Could you check a few things on this model? Use its own coordinates, in mm. Face numbers are marked on the shaded views. A direction names the side the tool comes from. Give positions to 0.01 mm unless a question says otherwise; leave off trailing zeros. Loops run counter-clockwise (first coordinate to the right, second up) from the corner with the lowest first, then second, coordinate; pieces in that order, holes last. Notation, with made-up numbers: (31, 28) -> (37, 28) arc R23 cw to (37, 62) -> close; hole circle Ø11 at (-7, 80.25). An arc over 180 degrees is marked (long way). Write each question's results on one line, items separated by ' | '. Start each with the question number.
Q1. If we section it at D-D, the plane x = 54.5: List the corners of the cut face in (y, z) for me, plus the area to 3 significant figures.
Q2. If we section it at A-A, the plane x = 0: List the corners of the cut face in (y, z) for me, plus the area to 3 significant figures.
Q3. If we section it at C-C, the plane y = 12: List the corners of the cut face in (x, z) for me.
Q4. If we section it at B-B, the plane z = -33: List the corners of the cut face in (x, y) for me.
Q5. Which directions (+Z, -Z, +X, -X, +Y, -Y) give clear straight access to the entire face, cutting with the end or side of a thin tool? Please do the marked faces 4, 5, 6 and 7.
Q6. Will these pins go through, and if not, where does the flat tip stop? P1, Ø11, axis at x = 1, z = 3, coming from the -Y side; P2, Ø1, axis at y = 19.5, z = -10.5, coming from the -X side; P3, Ø12, axis at y = 20.5, z = -5, coming from the +X side; P4, Ø4, axis at x = 1.5, z = -1.5, coming from the +Y side.
Q7. If I drill on line 1 along X through (y, z) = (41, 0); line 2 along Z through (x, y) = (55, 40.5); line 3 along Z through (x, y) = (57, 75), over which ranges is the centre line in solid material (lowest first)?
Q8. We'd pull the mould along Z, two halves only. Please class the marked faces 1, 2 and 3: released by +Z, released by -Z, zero draft, split by the parting line, or undercut.
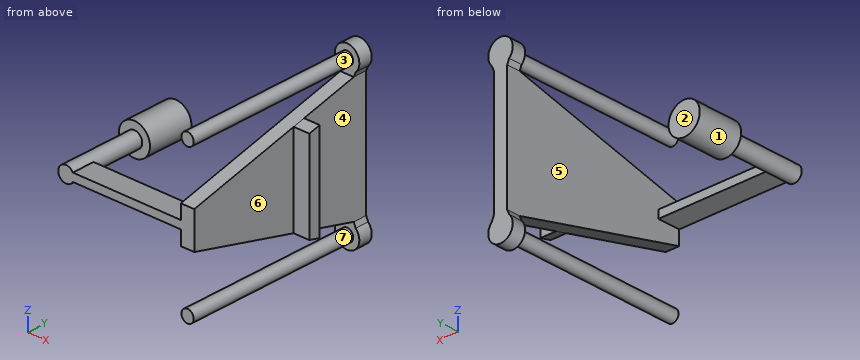
Autodesk Inventor part; units mm, degrees
ref_plane "YZ Plane" through (0, 0, 0) normal (1, 0, 0) x (0, 1, 0)
ref_plane "XZ Plane" through (0, 0, 0) normal (0, 1, 0) x (-1, 0, 0)
ref_plane "XY Plane" through (0, 0, 0) normal (0, 0, 1) x (1, 0, 0)
sketch "Sketch1" plane through (0, 0, 0) normal (0, 1, 0) x (-1, 0, 0)
  circle A0 centre (0, 0) radius 3.5
  dimension "d0" = 7
extrude "Extrusion1" add sketch "Sketch1" along normal blind 33
sketch "Sketch2" plane through (0, 33, 0) normal (0, 1, 0) x (1, 0, 0)
  circle A0 centre (0, 0) radius 7
  dimension "d3" = 14
extrude "Extrusion2" add sketch "Sketch2" along normal blind 20
sketch "Sketch3" plane through (0, 0, 0) normal (0, 0, 1) x (1, 0, 0)
  line L0 (0, 0) -> (57.5, 0)
  line L1 (57.5, 0) -> (57.5, 10)
  line L2 (57.5, 10) -> (0, 10)
  line L3 (0, 10) -> (0, 0)
  dimension "d6" = 57.5
  dimension "d7" = 10
extrude "Extrusion3" add sketch "Sketch3" along normal mid plane 3.5
sketch "Sketch4" plane through (57.5, 0, 1.75) normal (1, 0, 0) x (0, 0, -1)
  line L0 (1.75, 0) -> (9.75, 0)
  line L1 (9.75, 0) -> (28.75, 77)
  line L2 (1.75, 0) -> (1.75, 77)
  line L3 (1.75, 77) -> (28.75, 77)
  dimension "d10" = 8
  dimension "d11" = 27
  dimension "d12" = 77
extrude "Extrusion4" add sketch "Sketch4" against normal blind 6
sketch "Sketch5" plane through (57.5, 77, 0) normal (0, 1, 0) x (1, 0, 0)
  line L0 (0, 27) -> (0, 0)
  line L1 (0, 27) -> (-6, 27)
  line L2 (-6, 0) -> (-6, 27)
  line L3 (0, 0) -> (-6, 0)
  point P0 (-57.5, 0)
extrude "Extrusion5" add sketch "Sketch5" along normal blind 6
sketch "Sketch6" plane through (57.5, 83, 0) normal (0, 1, 0) x (1, 0, 0)
  circle A0 centre (-3, 33) radius 5.5
  line L0 (-6, 0) -> (0, 0)
  line L1 (-6, 27) -> (-6, 0)
  line L2 (-6, 27) -> (-8.5, 33)
  line L3 (0, 8) -> (0, 27)
  line L4 (0, 27) -> (2.5, 33)
  line L5 (0, 27) -> (-6, 27)
  line L6 (-6, 27) -> (0, 27)
  line L7 (-8.5, 33) -> (2.5, 33)
  point P0 (-57.5, 0)
  point P1 (0.8728, 29.0947)
  point P2 (-6.8728, 29.0947)
  dimension "d17" = 11
  dimension "d18" = 33
  dimension "d19" = 3
extrude "Extrusion6" add sketch "Sketch6" against normal blind 6
sketch "Sketch7" plane through (57.5, 77, 0) normal (0, -1, 0) x (1, 0, 0)
  arc A0 (-6.8728, -29.0947) -> (0.8728, -29.0947) centre (-3, -33) ccw
  circle A1 centre (-3, -33) radius 2.75
  point P0 (-57.5, 0)
  dimension "d22" = 5.5
extrude "Extrusion7" add sketch "Sketch7" along normal blind 77
mirror "Mirror1" about plane through (57.5, 0, 0) normal (0, 0, 1) of "Extrusion4", "Extrusion6", "Extrusion5", "Extrusion7"
sketch "Sketch8" plane through (57.5, 77, -27) normal (1, 0, 0) x (0, 0, -1)
  line L0 (-27, -77) -> (-27, -3.2697)
  line L1 (-46.8442, -29) -> (-7.1558, -29)
  line L2 (-7.1558, -29) -> (-5.9221, -24)
  line L3 (-5.9221, -24) -> (-48.0779, -24)
  line L4 (-48.0779, -24) -> (-46.8442, -29)
  line L5 (-46.8442, -29) -> (-5.9221, -24) construction
  line L6 (-7.1558, -29) -> (-48.0779, -24) construction
  line L7 (0, 6) -> (-54, 6)
  line L8 (-19, -77) -> (0, 0)
  line L9 (-35, -77) -> (-54, 0)
  point P0 (-27, -26.5754)
  dimension "d27" = 30
  dimension "d30" = 5
extrude "Extrusion8" add sketch "Sketch8" along normal blind 7
properties part number "Cube Cage" material "ABS Plastic"
Final values:
1) outline: (0, -35.75) -> (77, -35.75) -> (77, -38.5) -> (83, -38.5) -> (83, 38.5) -> (77, 38.5) -> (77, 35.75) -> (0, 35.75) -> (0, 30.25) -> (77, 30.25) -> (77, 27) -> (0, 8) -> (0, -8) -> (77, -27) -> (77, -30.25) -> (0, -30.25) -> close | area: 4,000 mm²
2) outline: (0, -3.5) -> (33, -3.5) -> (33, -7) -> (53, -7) -> (53, 7) -> (33, 7) -> (33, 3.5) -> (0, 3.5) -> close | area: 511 mm²
3) outline: circle Ø7 at (0, 0); (51.5, -10.96) -> (57.5, -10.96) -> (57.5, 10.96) -> (51.5, 10.96) -> close; circle Ø5.5 at (54.5, -33); circle Ø5.5 at (54.5, 33)
4) outline: (49, 77) -> (51.75, 77) -> (51.75, 0) -> (57.25, 0) -> (57.25, 77) -> (60, 77) -> (60, 83) -> (49, 83) -> close
5) face 4: +X, +Y | face 5: +Y | face 6: +Z, -Z, +X, -Y | face 7: -Y
6) P1: stops at y = 0 | P2: stops at x = 51.5 | P3: stops at x = 57.5 | P4: stops at y = 53
7) line 1: x = -7 to 7, 51.5 to 57.5 | line 2: z = -35.7 to -30.3, -17.99 to 17.99, 30.3 to 35.7 | line 3: z = -34.15 to -31.85, -26.51 to 26.51, 31.85 to 34.15
8) face 1: split by the parting line | face 2: zero draft | face 3: undercut
